```python
from build123d import *

# Parameters (mm, degrees)
BOSS_EXTRUDE1_DEPTH     = 10
SKETCH2_W               = 12
SKETCH2_H               = 20
BOSS_EXTRUDE2_DEPTH     = 40
SKETCH3_R               = 2.1
CUT_EXTRUDE1_DEPTH      = 86.29843199
CUT_EXTRUDE2_DEPTH      = 44
FILLET3_R               = 2
FILLET4_R               = 2
SKETCH6_R               = 2.6
CUT_EXTRUDE4_DEPTH      = 10
CUT_EXTRUDE5_DEPTH      = 5
CUT_EXTRUDE5_DEPTH_BACK = 5
SKETCH6_3_R             = 4.5
SKETCH6_3_R_2           = 2.6


with BuildPart() as part:
    # Sketch1 → Boss-Extrude1 (new body)
    with BuildSketch(Plane(origin=(0, 0, 0), x_dir=(1, 0, 0), z_dir=(0, 1, 0))):
        with BuildLine():
            Line((2, 0), (64.15, 0))
            ThreePointArc((64.15, 0), (65.564213562, 0.585786438), (66.15, 2))
            Line((66.15, 2), (66.15, 18))
            ThreePointArc((66.15, 18), (65.564213562, 19.414213562), (64.15, 20))
            Line((64.15, 20), (2, 20))
            ThreePointArc((2, 20), (0.585786438, 19.414213562), (0, 18))
            Line((0, 18), (0, 2))
            ThreePointArc((0, 2), (0.585786438, 0.585786438), (2, 0))
        make_face()
    extrude(amount=BOSS_EXTRUDE1_DEPTH)

    # Sketch2 → Boss-Extrude2 (add)
    with BuildSketch(Plane(origin=(0, 10, 0), x_dir=(1, 0, 0), z_dir=(0, 1, 0))):
        with Locations((6, 10)):
            Rectangle(SKETCH2_W, SKETCH2_H)
        with Locations((60.15, 10)):
            Rectangle(SKETCH2_W, SKETCH2_H)
    extrude(amount=BOSS_EXTRUDE2_DEPTH)

    # Sketch3 → Cut-Extrude1 (cut, through all)
    with BuildSketch(Plane(origin=(0, 50, 0), x_dir=(1, 0, 0), z_dir=(0, 1, 0))):
        with Locations(Location((6, 10, 0), (0, 0, 270))):
            Circle(SKETCH3_R)
        with Locations(Location((60.15, 10, 0), (0, 0, 270))):
            Circle(SKETCH3_R)
    extrude(amount=-CUT_EXTRUDE1_DEPTH, mode=Mode.SUBTRACT)

    # Sketch4 → Cut-Extrude2 (cut)
    with BuildSketch(Plane(origin=(0, 0, 0), x_dir=(-1, 0, 0), z_dir=(0, -1, 0))):
        Polygon((-8.121762239, 13.675), (-10.243524479, 10), (-8.121762239, 6.325), (-3.878237761, 6.325), (-1.756475521, 10), (-3.878237761, 13.675), align=None)
        Polygon((-62.271762239, 13.675), (-64.393524479, 10), (-62.271762239, 6.325), (-58.028237761, 6.325), (-55.906475521, 10), (-58.028237761, 13.675), align=None)
    extrude(amount=-CUT_EXTRUDE2_DEPTH, mode=Mode.SUBTRACT)

    # Fillet3
    fillet3_edges = [part.edges().sort_by_distance(p)[0] for p in [
        (0, 30, -20),
        (0, 30, 0),
        (66.15, 30, 0),
        (66.15, 30, -20),
    ]]
    fillet(fillet3_edges, radius=FILLET3_R)

    # Fillet4
    fillet4_edges = [part.edges().sort_by_distance(p)[0] for p in [
        (12, 10, -10),
        (54.15, 10, -10),
    ]]
    fillet(fillet4_edges, radius=FILLET4_R)

    # Sketch6 → Cut-Extrude4 (cut)
    with BuildSketch(Plane(origin=(0, 10, 0), x_dir=(1, 0, 0), z_dir=(0, 1, 0))):
        with Locations(Location((23.075, 10, 0), (0, 0, 270))):
            Circle(SKETCH6_R)
        with Locations(Location((43.075, 10, 0), (0, 0, 270))):
            Circle(SKETCH6_R)
    extrude(amount=-CUT_EXTRUDE4_DEPTH, mode=Mode.SUBTRACT)

    # Sketch6<3> → Cut-Extrude5 (cut, two sides: drawn at the far end of the back side and taken through both)
    # profile 1 of 2: a face of its own
    with BuildSketch(Plane(origin=(0, 10, 0), x_dir=(1, 0, 0), z_dir=(0, 1, 0)).offset(-CUT_EXTRUDE5_DEPTH_BACK)):
        with Locations(Location((43.075, 10, 0), (0, 0, 270))):
            Circle(SKETCH6_3_R)
        with Locations(Location((43.075, 10, 0), (0, 0, 270))):
            Circle(SKETCH6_3_R_2, mode=Mode.SUBTRACT)
    # profile 2 of 2: a face of its own
    with BuildSketch(Plane(origin=(0, 10, 0), x_dir=(1, 0, 0), z_dir=(0, 1, 0)).offset(-CUT_EXTRUDE5_DEPTH_BACK)):
        with Locations(Location((23.075, 10, 0), (0, 0, 270))):
            Circle(SKETCH6_3_R)
        with Locations(Location((23.075, 10, 0), (0, 0, 270))):
            Circle(SKETCH6_3_R_2, mode=Mode.SUBTRACT)
    extrude(amount=CUT_EXTRUDE5_DEPTH + CUT_EXTRUDE5_DEPTH_BACK, mode=Mode.SUBTRACT)


solid = part.part
```
Input: part model. Units: mm. Frame: model coordinates. A direction names the side the tool comes from. Coordinates: 2 decimals unless noted, no trailing zeros. Write each loop counter-clockwise with the first axis right and the second up, starting at its lowest first coordinate (ties: lowest second). Pieces come first, ordered by that corner, then holes. Notation, with made-up numbers: (40.25, 34.5) -> (87.25, 34.5) arc R11 cw to (87.25, 48.5) -> close; hole circle Ø4 at (18.25, -2). An arc over 180 degrees is marked (long way). Write each question's results on one line, items separated by ' | '.
Item 1: Material intervals for probe 1 along X at (y, z) = (47.1, -10); probe 2 along X at (y, z) = (2.35, -10) (3 decimals); probe 3 along X at (y, z) = (15, -18), sorted ascending.
Conclusion:
probe 1: x = 0 to 3.9, 8.1 to 12, 54.15 to 58.05, 62.25 to 66.15 | probe 2: x = 0 to 1.756, 10.244 to 20.475, 25.675 to 40.475, 45.675 to 55.906, 64.394 to 66.15 | probe 3: x = 0 to 12, 54.15 to 66.15
Item 2: Pin query (flat end, axial travel): pin 1 Ø4 at (x, y) = (12.5, 19.5) entering from -Z; pin 2 Ø5 at (x, z) = (60.15, -10) entering from -Y; pin 3 Ø4 at (x, z) = (32, -13.5) entering from +Y. Return the tip coordinate at first contact, or that it passes through.
Conclusion:
pin 1: stops at z = -20 | pin 2: stops at y = 44 | pin 3: stops at y = 10
Item 3: Set-up query: faces 5 (the cylindrical face through (0.57, 30.28, -19.4)), 6 (the flat face through (12, 31, -10)), 7 (the flat face through (63.32, 21.69, -11.86)). Return all of +Z, -Z, +X, -X, +Y, -Y with unobstructed straight access to the full face (end or side cutting, diameter ignored); none if empty.
Conclusion:
face 5: -Z, -X, +Y, -Y | face 6: +Z, -Z, +Y | face 7: -Y
Item 4: Section query A-A on y = 18.5. Return loops of the section in (x, z) (3 decimals).
Conclusion:
outline: (0, -18) arc R2 ccw to (2, -20) -> (12, -20) -> (12, 0) -> (2, 0) arc R2 ccw to (0, -2) -> close; (54.15, -20) -> (64.15, -20) arc R2 ccw to (66.15, -18) -> (66.15, -2) arc R2 ccw to (64.15, 0) -> (54.15, 0) -> close; hole (1.756, -10) -> (3.878, -13.675) -> (8.122, -13.675) -> (10.244, -10) -> (8.122, -6.325) -> (3.878, -6.325) -> close; hole (55.906, -10) -> (58.028, -13.675) -> (62.272, -13.675) -> (64.394, -10) -> (62.272, -6.325) -> (58.028, -6.325) -> close
Item 5: Mould query, pull axis X, two halves, no side actions, for faces 1 (the flat face through (5.9, 50, -12.4)), 2 (the cylindrical face through (65.55, 4.93, -0.57)), 3 (the cylindrical face through (20.537, 2.535, -10.564)), 4 (the cylindrical face through (0.57, 4.93, -0.6)). Classes: +X half, -X half, draft (parallel to the pull), parting line (faces both ways), or undercut.
Conclusion:
face 1: draft | face 2: +X half | face 3: undercut | face 4: -X half
Item 6: Section query C-C on x = 16. Return loops of the section in (y, z).
Conclusion:
outline: (0, -20) -> (10, -20) -> (10, 0) -> (0, 0) -> close
Item 7: Section query B-B on x = 60.15. Return loops of the section in (y, z) (3 decimals).
Conclusion:
outline: (0, -20) -> (50, -20) -> (50, -12.1) -> (44, -12.1) -> (44, -13.675) -> (0, -13.675) -> close; (0, -6.325) -> (44, -6.325) -> (44, -7.9) -> (50, -7.9) -> (50, 0) -> (0, 0) -> close
